Print and shaded views of the part. All mm, measured from the part's lowest x, y and z. Round coordinates to 2 decimals unless told otherwise and drop trailing zeros. Write each loop counter-clockwise with the first axis right and the second up, starting at its lowest first coordinate (ties: lowest second). Pieces come first, ordered by that corner, then holes. Notation, with made-up numbers: (74.25, -14.75) -> (121.25, -14.75) arc R22 ccw to (121.25, 1.25) -> close; hole circle Ø9 at (14, 11.25). An arc over 180 degrees is marked (long way). Return JSON: item names as keys, results as strings. Group by question number.
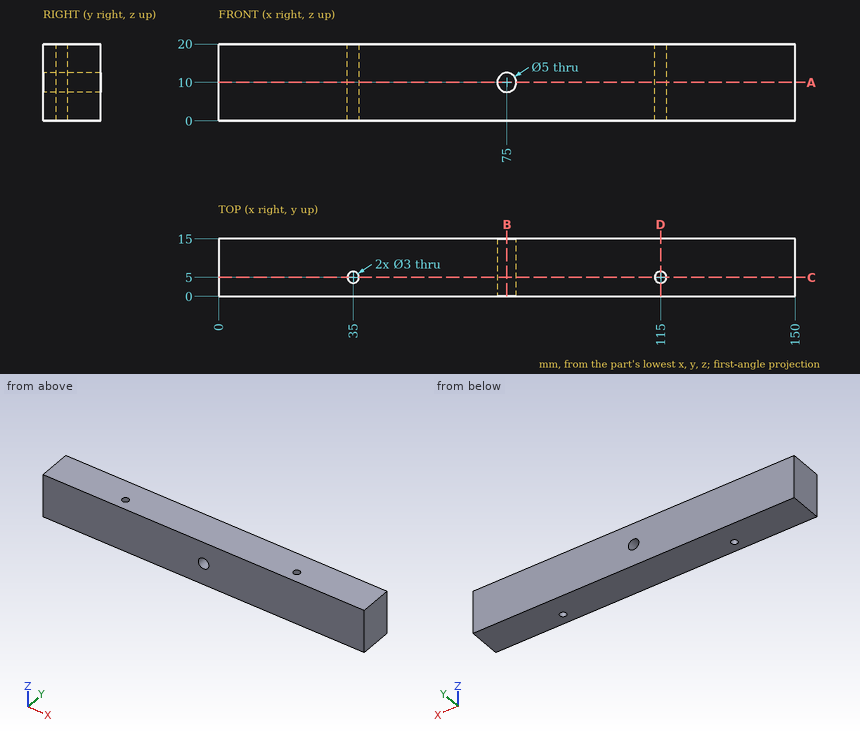
Item 1: Cut at D-D (x = 115). Write the cut outline in (y, z), then the cut area to 3 significant figures.
Item 2: Cut at A-A (z = 10). Write the cut outline in (x, y), then the cut area to 3 significant figures.
Item 3: Cut at C-C (y = 5). Write the cut outline in (x, z), then the cut area to 3 significant figures.
Item 4: Wall check: L1, parallel to Z at x = 75, y = 5.75; L2, parallel to X at y = 5.5, z = 19; L3, parallel to Y at x = 35, z = 5. Give the ranges that are in metal, low to high.
Item 5: Cut at B-B (x = 75). Write the cut outline in (y, z).
Checks:
{
 "1": {"outline": "(0, 0) -> (3.5, 0) -> (3.5, 20) -> (0, 20) -> close; (6.5, 0) -> (15, 0) -> (15, 20) -> (6.5, 20) -> close", "area": "240 mm2"},
 "2": {"outline": "(0, 0) -> (72.5, 0) -> (72.5, 15) -> (0, 15) -> close; (77.5, 0) -> (150, 0) -> (150, 15) -> (77.5, 15) -> close; hole circle Ø3 at (35, 5); hole circle Ø3 at (115, 5)", "area": "2,160 mm2"},
 "3": {"outline": "(0, 0) -> (33.5, 0) -> (33.5, 20) -> (0, 20) -> close; (36.5, 0) -> (113.5, 0) -> (113.5, 20) -> (36.5, 20) -> close; (116.5, 0) -> (150, 0) -> (150, 20) -> (116.5, 20) -> close; hole circle Ø5 at (75, 10)", "area": "2,860 mm2"},
 "4": {"L1": "z = 0 to 7.5, 12.5 to 20", "L2": "x = 0 to 33.59, 36.41 to 113.59, 116.41 to 150", "L3": "y = 0 to 3.5, 6.5 to 15"},
 "5": {"outline": "(0, 0) -> (15, 0) -> (15, 7.5) -> (0, 7.5) -> close; (0, 12.5) -> (15, 12.5) -> (15, 20) -> (0, 20) -> close"}
}
